from build123d import *

# Parameters (mm, degrees)
F1_DEPTH = 2.794
F2_DEPTH = 1.27
F4_DEPTH = 2.54
F6_DEPTH = 2.54
F8_DEPTH = 2.54
F9_R     = 2.54
F10_R    = 1.52399
F11_R    = 1.27
F12_R    = 1.26999


# Not quite as in the source:
# - a fillet or chamfer is up to 0.001 mm smaller than in the source, because OpenCascade refuses the exact size


with BuildPart() as f1:
    # F0 (on Top) → F1 (new body, symmetric)
    with BuildSketch(Plane.XY):
        with BuildLine():
            Line((13.4556421247, 40.506048555), (-29.0893578753, 40.506048555))
            ThreePointArc((-29.0893578753, 40.506048555), (-32.6881934203, 39.8473107196), (-35.8203578753, 37.9565175945))
            Line((-35.8203578753, 37.9565175945), (-35.8203578753, 30.346048555))
            ThreePointArc((-35.8203578753, 30.346048555), (-33.8488936195, 35.1055842992), (-29.0893578753, 37.077048555))
            Line((-29.0893578753, 37.077048555), (13.4556421247, 37.077048555))
            ThreePointArc((13.4556421247, 37.077048555), (18.2151778689, 35.1055842992), (20.1866421247, 30.346048555))
            Line((20.1866421247, 30.346048555), (20.1866421247, 37.9565175945))
            ThreePointArc((20.1866421247, 37.9565175945), (17.0544776697, 39.8473107196), (13.4556421247, 40.506048555))
        make_face()
        with BuildLine():
            ThreePointArc((-29.0893578753, 37.077048555), (-33.8488936195, 35.1055842992), (-35.8203578753, 30.346048555))
            Line((-35.8203578753, 30.346048555), (-35.8203578753, -43.313951445))
            ThreePointArc((-35.8203578753, -43.313951445), (-33.8488936195, -48.0734871891), (-29.0893578753, -50.044951445))
            Line((-29.0893578753, -50.044951445), (13.4556421247, -50.044951445))
            ThreePointArc((13.4556421247, -50.044951445), (18.2151778689, -48.0734871891), (20.1866421247, -43.313951445))
            Line((20.1866421247, -43.313951445), (20.1866421247, 30.346048555))
            ThreePointArc((20.1866421247, 30.346048555), (18.2151778689, 35.1055842992), (13.4556421247, 37.077048555))
            Line((13.4556421247, 37.077048555), (-29.0893578753, 37.077048555))
        make_face()
        with BuildLine():
            Line((-35.8203578753, 30.346048555), (-35.8203578753, 37.9565175945))
            ThreePointArc((-35.8203578753, 37.9565175945), (-38.3525257999, 34.5196944432), (-39.2493578753, 30.346048555))
            Line((-39.2493578753, 30.346048555), (-39.2493578753, -43.313951445))
            ThreePointArc((-39.2493578753, -43.313951445), (-36.2735627721, -50.4981563418), (-29.0893578753, -53.473951445))
            Line((-29.0893578753, -53.473951445), (13.4556421247, -53.473951445))
            ThreePointArc((13.4556421247, -53.473951445), (20.6398470216, -50.4981563418), (23.6156421247, -43.313951445))
            Line((23.6156421247, -43.313951445), (23.6156421247, 30.346048555))
            ThreePointArc((23.6156421247, 30.346048555), (22.7188100493, 34.5196944432), (20.1866421247, 37.9565175945))
            Line((20.1866421247, 37.9565175945), (20.1866421247, 30.346048555))
            Line((20.1866421247, 30.346048555), (20.1866421247, -43.313951445))
            ThreePointArc((20.1866421247, -43.313951445), (18.2151778689, -48.0734871891), (13.4556421247, -50.044951445))
            Line((13.4556421247, -50.044951445), (-29.0893578753, -50.044951445))
            ThreePointArc((-29.0893578753, -50.044951445), (-33.8488936195, -48.0734871891), (-35.8203578753, -43.313951445))
            Line((-35.8203578753, -43.313951445), (-35.8203578753, 30.346048555))
        make_face()
    extrude(amount=F1_DEPTH, both=True)

    # F0 (on Top) → F2 (cut, symmetric)
    with BuildSketch(Plane.XY):
        with BuildLine():
            Line((13.4556421247, 40.506048555), (-29.0893578753, 40.506048555))
            ThreePointArc((-29.0893578753, 40.506048555), (-32.6881934203, 39.8473107196), (-35.8203578753, 37.9565175945))
            Line((-35.8203578753, 37.9565175945), (-35.8203578753, 30.346048555))
            ThreePointArc((-35.8203578753, 30.346048555), (-33.8488936195, 35.1055842992), (-29.0893578753, 37.077048555))
            Line((-29.0893578753, 37.077048555), (13.4556421247, 37.077048555))
            ThreePointArc((13.4556421247, 37.077048555), (18.2151778689, 35.1055842992), (20.1866421247, 30.346048555))
            Line((20.1866421247, 30.346048555), (20.1866421247, 37.9565175945))
            ThreePointArc((20.1866421247, 37.9565175945), (17.0544776697, 39.8473107196), (13.4556421247, 40.506048555))
        make_face()
        with BuildLine():
            ThreePointArc((-29.0893578753, 37.077048555), (-33.8488936195, 35.1055842992), (-35.8203578753, 30.346048555))
            Line((-35.8203578753, 30.346048555), (-35.8203578753, -43.313951445))
            ThreePointArc((-35.8203578753, -43.313951445), (-33.8488936195, -48.0734871891), (-29.0893578753, -50.044951445))
            Line((-29.0893578753, -50.044951445), (13.4556421247, -50.044951445))
            ThreePointArc((13.4556421247, -50.044951445), (18.2151778689, -48.0734871891), (20.1866421247, -43.313951445))
            Line((20.1866421247, -43.313951445), (20.1866421247, 30.346048555))
            ThreePointArc((20.1866421247, 30.346048555), (18.2151778689, 35.1055842992), (13.4556421247, 37.077048555))
            Line((13.4556421247, 37.077048555), (-29.0893578753, 37.077048555))
        make_face()
    extrude(amount=F2_DEPTH, both=True, mode=Mode.SUBTRACT)

    # F3 (on face) → F4 (cut)
    with BuildSketch(Plane.XY.offset(2.794)):
        Polygon((-16.199497506, 18.9658571035), (-25.0740814954, 18.9658571035), (-25.0740814954, -30.413236469), (-16.199497506, -30.413236469), (-16.199497506, -16.4083634515), (-12.8775097826, -11.8783802343), (1.1254162528, -30.413236469), (12.8968711942, -30.413236469), (-7.0793794499, -3.9718389452), (9.7415978089, 18.9658571035), (-1.1809705757, 18.9658571035), (-16.199497506, -1.5139521565), align=None)
    extrude(amount=-F4_DEPTH, mode=Mode.SUBTRACT)

    # F5 (on face) → F6 (cut)
    with BuildSketch(Plane(origin=(0, 0, -2.794), x_dir=(1, 0, 0), z_dir=(0, 0, -1))):
        with BuildLine():
            Line((-29.1631240398, 40.1679472998), (-29.1631240398, -27.4539431557))
            ThreePointArc((-29.1631240398, -27.4539431557), (-23.7097460777, -32.9073211178), (-18.2563681155, -27.4539431557))
            Line((-18.2563681155, -27.4539431557), (-18.2563681155, 40.1679472998))
            ThreePointArc((-18.2563681155, 40.1679472998), (-23.7097460777, 45.6213252619), (-29.1631240398, 40.1679472998))
        make_face()
        with BuildLine():
            ThreePointArc((-5.0461939536, -35.2972820401), (-3.9444430731, -34.1955311596), (-5.0461939536, -33.0937802792))
            Line((-5.0461939536, -33.0937802792), (-10.8487373218, -33.0937802792))
            ThreePointArc((-10.8487373218, -33.0937802792), (-11.9504882023, -34.1955311596), (-10.8487373218, -35.2972820401))
            Line((-10.8487373218, -35.2972820401), (-5.0461939536, -35.2972820401))
        make_face()
    extrude(amount=-F6_DEPTH, mode=Mode.SUBTRACT)

    # F7 (on face) → F8 (cut)
    with BuildSketch(Plane.XY.offset(2.794)):
        with BuildLine():
            Line((1.8508417322, 40.506048555), (-17.466821873, 40.506048555))
            ThreePointArc((-17.466821873, 40.506048555), (-7.8079900704, 31.0812084526), (1.8508417322, 40.506048555))
        make_face()
    extrude(amount=-F8_DEPTH, mode=Mode.SUBTRACT)

    # F9
    f9_edges = [f1.edges().sort_by_distance(p)[0] for p in [
        (1.850842, 40.506049, 2.032),
        (-17.466822, 40.506049, 2.032),
    ]]
    fillet(f9_edges, radius=F9_R)

    # F10 (radius 1.524 in the source; OpenCascade refuses exactly that, so slightly less here)
    f10_edges = [f1.edges().sort_by_distance(p)[0] for p in [
        (-39.249358, -6.483951, 2.794),
        (-39.249358, -6.483951, -2.794),
        (-29.163124, -6.357002, -2.794),
    ]]
    fillet(f10_edges, radius=F10_R)

    # F11
    f11_edges = [f1.edges().sort_by_distance(p)[0] for p in [
        (9.741598, 18.965857, 2.032),
        (-1.180971, 18.965857, 2.032),
        (-16.199498, 18.965857, 2.032),
        (-16.199498, -1.513952, 2.032),
        (-7.079379, -3.971839, 2.032),
        (12.896871, -30.413236, 2.032),
        (1.125416, -30.413236, 2.032),
        (-12.87751, -11.87838, 2.032),
        (-16.199498, -16.408363, 2.032),
        (-16.199498, -30.413236, 2.032),
        (-25.074081, -30.413236, 2.032),
        (-25.074081, 18.965857, 2.032),
    ]]
    fillet(f11_edges, radius=F11_R)

    # F12 (radius 1.27 in the source; OpenCascade refuses exactly that, so slightly less here)
    f12_edges = [f1.edges().sort_by_distance(p)[0] for p in [
        (-35.820358, -2.678717, 1.27),
        (-35.820358, -2.678717, -1.27),
    ]]
    fillet(f12_edges, radius=F12_R)


solid = f1.part
Work out the finished part from the listing and answer in its coordinate system (mm). A direction names the side the tool comes from. Give positions to 0.01 mm unless a question says otherwise; leave off trailing zeros. One line per item, written item: value. Start each with the question number.
1. Find section A-A (y = -22.5). State how many separate pieces and enclosed holes the cut face has, then the cut area to 3 significant figures.
2. For a pull along Y with two mould halves and no side action, classify faces 1 (the flat face through (-39.249, -6, 0)), 2 (the flat face through (-14.93, -14.68, 2.04)), 3 (the cylindrical face through (-38.25, 34.74, 0.02)) as +Y half, -Y half, draft (parallel to the pull), parting line (faces both ways), or undercut.
3. Consider probe 1 along Z at (x, y) = (9.5, -39.5); probe 2 along X at (y, z) = (-11, 0.2); probe 3 along Y at (x, z) = (-5, 2.6). Determine where each line is inside the solid, lowest interval first.
4. For faces 4 (the cylindrical face through (-36.35, -50.42, 0.02)), 5 (the flat face through (-5.64, -21.46, 2.04)), 6 (the flat face through (-2, -4, 1.27)), determine the directions among +Z, -Z, +X, -X, +Y, -Y from which every point of the face is accessible in a straight line to the end or side of a thin tool.
5. Given pin 1 (0.5 mm diameter, centred on y = 6, z = 2, fed in from +X); pin 2 (0.5 mm diameter, centred on x = -21.5, z = 2, fed in from -Y); pin 3 (0.8 mm diameter, centred on x = 4.5, z = 2, fed in from +Y); pin 4 (1.5 mm diameter, centred on x = -21, y = -25, fed in from +Z) (3 decimals), each flat-ended and moving along its own axis, determine where each tip first touches the part or whether it passes through.
Geometry results:
1. separate pieces: 3
1. enclosed holes: 0
1. area: 159 mm2
2. face 1: draft
2. face 2: undercut
2. face 3: +Y half
3. probe 1: -2.79 to -1.27, 1.27 to 2.79
3. probe 2: -39.25 to -35.8, 20.17 to 23.62
3. probe 3: -52.69 to -22.31, -6.72 to -1.14, 13.76 to 30.69
4. face 4: +Z, -Z, -X, -Y
4. face 5: +Z
4. face 6: +Y
5. pin 1: x = 23.54
5. pin 2: y = -53.4
5. pin 3: y = 40.47
5. pin 4: through
